```python
from build123d import *

# Parameters (mm, degrees)
SKETCH_1_W          = 60
SKETCH_1_H          = 55
SKETCH_1_R          = 20
EXTRUDE_1_DEPTH     = 2
SKETCH_2_W          = 60
SKETCH_2_H          = 55
SKETCH_2_W_2        = 56
SKETCH_2_H_2        = 51
EXTRUDE_2_DEPTH     = 48
CUT_EXTRUDE_1_REACH = 96.493
CUT_EXTRUDE_2_REACH = 96.493
FILLET_1_R          = 2


with BuildPart() as part:
    # 草图1 → 凸台-拉伸1 (new body)
    with BuildSketch(Plane.XY):
        with Locations((30, -27.5)):
            Rectangle(SKETCH_1_W, SKETCH_1_H)
        with Locations((30, -26)):
            Circle(SKETCH_1_R, mode=Mode.SUBTRACT)
    extrude(amount=EXTRUDE_1_DEPTH)

    # 草图2 → 凸台-拉伸2 (add)
    with BuildSketch(Plane(origin=(0, 0, 0), x_dir=(-1, 0, 0), z_dir=(0, 0, -1))):
        with Locations((-30, -27.5)):
            Rectangle(SKETCH_2_W, SKETCH_2_H)
        with Locations((-30, -27.5)):
            Rectangle(SKETCH_2_W_2, SKETCH_2_H_2, mode=Mode.SUBTRACT)
    extrude(amount=EXTRUDE_2_DEPTH)

    # 切除-拉伸1: up to this face of the body (flat: up to its plane)
    cut_extrude_1_end = Plane(part.part.faces().sort_by_distance((30, 0, -23))[0])
    # 草图3 → 切除-拉伸1 (cut, up to the picked face)
    with BuildSketch(Plane.XZ.offset(55), mode=Mode.PRIVATE) as cut_extrude_1_sk1:
        with BuildLine():
            Line((30, -48), (4, -48))
            Line((4, -48), (4, -30))
            ThreePointArc((4, -30), (30, -4), (56, -30))
            Line((56, -30), (56, -48))
            Line((56, -48), (30, -48))
        make_face()
    cut_extrude_1_tool1 = split(extrude(cut_extrude_1_sk1.sketch, amount=-CUT_EXTRUDE_1_REACH, mode=Mode.PRIVATE), bisect_by=cut_extrude_1_end, keep=Keep.BOTH, mode=Mode.PRIVATE)
    add(cut_extrude_1_tool1.solids().sort_by(Axis((30, -55, -28.351568), (0, 1, 0)))[0], mode=Mode.SUBTRACT)

    # 切除-拉伸2: up to this face of the body (flat: up to its plane)
    cut_extrude_2_end = Plane(part.part.faces().sort_by_distance((60, -27.5, -23))[0])
    # 草图4 → 切除-拉伸2 (cut, up to the picked face)
    with BuildSketch(Plane.ZY, mode=Mode.PRIVATE) as cut_extrude_2_sk1:
        with BuildLine():
            Line((-26, -7), (-48, -7))
            Line((-48, -7), (-48, -48))
            Line((-48, -48), (-26, -48))
            ThreePointArc((-26, -48), (-5.5, -27.5), (-26, -7))
        make_face()
    cut_extrude_2_tool1 = split(extrude(cut_extrude_2_sk1.sketch, amount=-CUT_EXTRUDE_2_REACH, mode=Mode.PRIVATE), bisect_by=cut_extrude_2_end, keep=Keep.BOTH, mode=Mode.PRIVATE)
    add(cut_extrude_2_tool1.solids().sort_by(Axis((0, -27.5, -28.674932), (1, 0, 0)))[0], mode=Mode.SUBTRACT)

    # 圆角1
    fillet_1_edges = [part.edges().sort_by_distance(p)[0] for p in [
        (56, 0, -39),
        (58, 0, -48),
        (2, 0, -48),
        (4, 0, -39),
        (30, 0, -4),
        (0, -7, -37),
        (0, -3.5, -48),
        (0, 0, -23),
        (0, -51.5, -48),
        (0, -48, -37),
        (0, -27.5, -5.5),
        (10, -26, 2),
        (30, 0, 2),
        (0, -27.5, 2),
        (60, -27.5, 2),
        (60, 0, -23),
        (60, -3.5, -48),
        (60, -7, -37),
        (60, -27.5, -5.5),
        (60, -48, -37),
        (60, -51.5, -48),
        (0, -55, -23),
        (30, -55, 2),
        (60, -55, -23),
        (58, -55, -48),
        (56, -55, -39),
        (30, -55, -4),
        (4, -55, -39),
        (2, -55, -48),
    ]]
    fillet(fillet_1_edges, radius=FILLET_1_R - 0.0001)  # a hair under: the kernel refuses the full size


solid = part.part
```
Could you check a few things on this model? Use its own coordinates, in mm. A direction names the side the tool comes from. Coordinates: 2 decimals unless noted, no trailing zeros. Write item = value, one per line. Start each with the question number.
(1) Which directions (+Z, -Z, +X, -X, +Y, -Y) give clear straight access to the entire face, cutting with the end or side of a thin tool? Please do faces 1 (the face through (59.43, -48.6, -36.85)), 2 (the face through (57.2, -0.8, -47.6)), 3 (the face through (0.57, -48.6, -36.85)), 4 (the face through (56.6, -0.57, -39.13)), 5 (the face through (3.4, -54.43, -38.87)).
(2) I want a section at B-B (z = -41). Give the number of separate pieces and of enclosed holes in the cut face, plus the area to 3 significant figures.
(3) Will these pins go through, and if not, where does the flat tip stop? pin 1 (8 mm diameter, centred on x = 53, y = -48.5, fed in from -Z); pin 2 (8 mm diameter, centred on y = -49, z = -20.5, fed in from +X); pin 3 (12 mm diameter, centred on x = 22.5, z = -10, fed in from -Y).
(4) We'd pull the mould along X, two halves only. Please class faces 6 (the face through (30.39, -54.43, 1.4)), 7 (the face through (34, -2, -4)), 8 (the face through (58, -28, -2)), 9 (the face through (59.43, -3.91, -47.4)): released by +X, released by -X, zero draft, split by the parting line, or undercut.
(5) I need wall thicknesses on line 1 (X direction, y = -7.5, z = -10.5); line 2 (Y direction, x = 30, z = 0.05); line 3 (Z direction, x = 54, y = -5.5). Which ranges of each line are inside material? Lowest first, please. Write a range as [from, to].
Result set:
q1.face_1 = -Z, +X
q1.face_2 = -Z, +X, -X, +Y
q1.face_3 = -Z, -X
q1.face_4 = -Z, +Y
q1.face_5 = -Z, -Y
q2.separate_pieces = 4
q2.enclosed_holes = 0
q2.area = 61.7 mm2
q3.pin_1 = 0
q3.pin_2 = 60
q3.pin_3 = -54.89
q4.face_6 = zero draft
q4.face_7 = undercut
q4.face_8 = undercut
q4.face_9 = released by +X
q5.line_1 = [0, 2], [58, 60]
q5.line_2 = [-55, -46], [-6, 0]
q5.line_3 = [0, 2]
